from build123d import *

# Parameters (mm, degrees)
EXTRUDE_1_DEPTH     = 275
SKETCH_2_R          = 3
SKETCH_2_R_2        = 2
CUT_EXTRUDE_1_DEPTH = 279.25348156


with BuildPart() as part:
    # 草图1 → 凸台-拉伸1 (new, symmetric)
    with BuildSketch(Plane(origin=(0, 0, 0), x_dir=(1, 0, 0), z_dir=(0, 1, 0))):
        with BuildLine():
            Line((4, 0), (26, 0))
            ThreePointArc((26, 0), (28.828427125, 1.171572875), (30, 4))
            Line((30, 4), (30, 26))
            ThreePointArc((30, 26), (28.828427125, 28.828427125), (26, 30))
            Line((26, 30), (4, 30))
            ThreePointArc((4, 30), (1.171572875, 28.828427125), (0, 26))
            Line((0, 26), (0, 4))
            ThreePointArc((0, 4), (1.171572875, 1.171572875), (4, 0))
        make_face()
        with BuildLine():
            Line((4, 2), (26, 2))
            ThreePointArc((26, 2), (27.414213562, 2.585786438), (28, 4))
            Line((28, 4), (28, 26))
            ThreePointArc((28, 26), (27.414213562, 27.414213562), (26, 28))
            Line((26, 28), (4, 28))
            ThreePointArc((4, 28), (2.585786438, 27.414213562), (2, 26))
            Line((2, 26), (2, 4))
            ThreePointArc((2, 4), (2.585786438, 2.585786438), (4, 2))
        make_face(mode=Mode.SUBTRACT)
    extrude(amount=EXTRUDE_1_DEPTH, both=True)

    # 草图2 → 切除-拉伸1 (cut, through all)
    with BuildSketch(Plane.XY):
        with Locations((18.5, 234)):
            Circle(SKETCH_2_R)
        with Locations((18.5, 200)):
            Circle(SKETCH_2_R)
        with Locations((18.5, -200)):
            Circle(SKETCH_2_R)
        with Locations((18.5, -234)):
            Circle(SKETCH_2_R)
        with Locations((15, 265)):
            Circle(SKETCH_2_R_2)
        with Locations((15, 100)):
            Circle(SKETCH_2_R_2)
        with Locations((15, -100)):
            Circle(SKETCH_2_R_2)
        with Locations((15, -265)):
            Circle(SKETCH_2_R_2)
    extrude(amount=-CUT_EXTRUDE_1_DEPTH, mode=Mode.SUBTRACT)


solid = part.part
Input: part model. Units: mm. Frame: model coordinates. A direction names the side the tool comes from. Round coordinates to 2 decimals unless told otherwise and drop trailing zeros. Order: outer loops, then holes, each group sorted by start corner. A loop starts at its lowest first (then second) coordinate and runs counter-clockwise, first axis right, second up.
1. Material intervals for line 1 (Y direction, x = 18.5, z = -28.7); line 2 (Z direction, x = 19.5, y = 100.5); line 3 (X direction, y = 193.5, z = -23.75), sorted ascending.
The answers:
line 1: y = -275 to -237, -231 to -203, -197 to 197, 203 to 231, 237 to 275
line 2: z = -30 to -28, -2 to 0
line 3: x = 0 to 2, 28 to 30
2. Cut plane A-A, the plane z = -12. Output: boundary loops of the cut face in (x, y).
The answers:
outline: (0, -275) - (2, -275) - (2, 275) - (0, 275) - close; (28, -275) - (30, -275) - (30, 275) - (28, 275) - close
3. Cut plane B-B, the plane y = -162.5. Output: boundary loops of the cut face in (x, z).
The answers:
outline: (0, -26) arc R4 ccw to (4, -30) - (26, -30) arc R4 ccw to (30, -26) - (30, -4) arc R4 ccw to (26, 0) - (4, 0) arc R4 ccw to (0, -4) - close; hole (2, -26) arc R2 ccw to (4, -28) - (26, -28) arc R2 ccw to (28, -26) - (28, -4) arc R2 ccw to (26, -2) - (4, -2) arc R2 ccw to (2, -4) - close
4. Mould query, pull axis Z, two halves, no side actions, for faces 1 (the face through (15, 4, -30)), 2 (the face through (2, 4, -15)), 3 (the face through (1, 275, -15)). Classes: released by +Z, released by -Z, zero draft, split by the parting line, or undercut.
The answers:
face 1: released by -Z
face 2: undercut
face 3: zero draft
5. Set-up query: faces 4 (the face through (1, -275, -15)), 5 (the face through (28, 4, -15)). Return all of +Z, -Z, +X, -X, +Y, -Y with unobstructed straight access to the full face (end or side cutting, diameter ignored); none if empty.
The answers:
face 4: +Z, -Z, +X, -X, -Y
face 5: +Y, -Y
